```python
from build123d import *

# Parameters (mm, degrees)
SKETCH1_W           = 28
SKETCH1_H           = 78
BOSS_EXTRUDE1_DEPTH = 58
CUT_EXTRUDE1_DEPTH  = 10
CUT_EXTRUDE2_DEPTH  = 20
CUT_EXTRUDE3_DEPTH  = 30
SKETCH5_R           = 2.75
BOSS_EXTRUDE2_DEPTH = 6


with BuildPart() as part:
    # Sketch1 → Boss-Extrude1 (new body)
    with BuildSketch(Plane(origin=(0, 0, 0), x_dir=(1, 0, 0), z_dir=(0, 1, 0))):
        Rectangle(SKETCH1_W, SKETCH1_H)
    extrude(amount=BOSS_EXTRUDE1_DEPTH)

    # Sketch2 → Cut-Extrude1 (cut)
    with BuildSketch(Plane(origin=(14, 0, 0), x_dir=(0, 0, -1), z_dir=(1, 0, 0))):
        Polygon((-39, 8), (-14.181832949, 8), (9.133549959, 58), (-39, 58), align=None)
    extrude(amount=-CUT_EXTRUDE1_DEPTH, mode=Mode.SUBTRACT)

    # Sketch3 → Cut-Extrude2 (cut)
    with BuildSketch(Plane(origin=(4, 0, 0), x_dir=(0, 0, -1), z_dir=(1, 0, 0))):
        Polygon((-39, 16), (-15, 16), (-15, 40.557545824), (1, 40.557545824), (9.133549959, 58), (-39, 58), align=None)
    extrude(amount=-CUT_EXTRUDE2_DEPTH, mode=Mode.SUBTRACT)

    # Sketch4 → Cut-Extrude3 (cut)
    with BuildSketch(Plane(origin=(14, 0, 0), x_dir=(0, 0, -1), z_dir=(1, 0, 0))):
        Polygon((9.133549959, 58), (22.517676281, 52.154545261), (8.109098298, 19.163745323), (12.691153845, 17.162553937), (27.099731828, 50.153353874), (39, 44.95596726), (39, 58), align=None)
    extrude(amount=-CUT_EXTRUDE3_DEPTH, mode=Mode.SUBTRACT)

    # Sketch5 → Boss-Extrude2 (add)
    with BuildSketch(Plane(origin=(0, 52.058969702, -22.736512182), x_dir=(1, 0, 0), z_dir=(0, 0.9164111093707628, -0.40023827730721606))):
        with Locations(Location((-8.021015767, -7.343733433, 0), (0, 0, 90))):
            Circle(SKETCH5_R)
        with Locations(Location((6.818441056, -7.343733433, 0), (0, 0, 90))):
            Circle(SKETCH5_R)
    extrude(amount=BOSS_EXTRUDE2_DEPTH)


solid = part.part
```
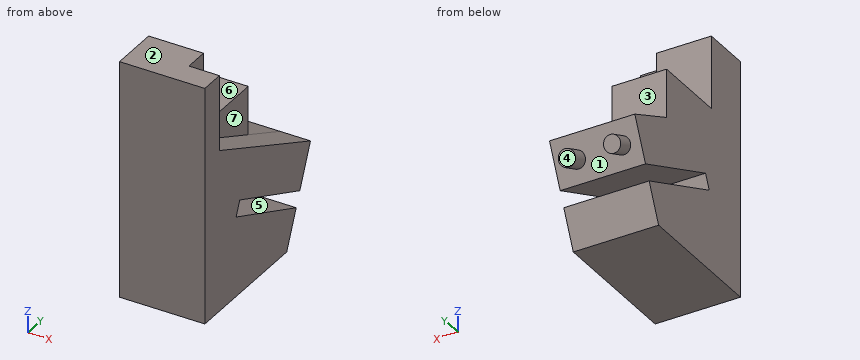
Geometry check sheet. Reference: the model listing, model coordinates, mm. Face numbers are marked on the shaded views. A direction names the side the tool comes from. Coordinates: 2 decimals unless noted, no trailing zeros. Loops run counter-clockwise (first coordinate to the right, second up) from the corner with the lowest first, then second, coordinate; pieces in that order, holes last. Notation, with made-up numbers: (0, -14) - (52, -14) arc R17 cw to (52, -6) - close; hole circle Ø1 at (62.5, -32). An arc over 180 degrees is marked (long way). One line per item, written item: value. Start each with the question number.
(1) Depth check by flat-ended pin: P1, Ø6, axis at x = 9, y = 52, coming from the -Z side; P2, Ø1, axis at x = -2, y = 38, coming from the +Z side; P3, Ø11, axis at x = 8.5, z = 31, coming from the +Y side. Enter the tip coordinate at first touch or a pass-through.
(2) Cross-section at C-C on x = -0.5. Enter the section's corners in (y, z), plus the area to 3 significant figures.
(3) Cross-section at D-D on y = 39. Enter the section's corners in (x, z), plus the area to 3 significant figures.
(4) Mould release check, pull along Z, two halves, no side actions. Record for the marked faces 1, 2, 3 and 4: released by +Z, released by -Z, zero draft, split by the parting line, or undercut.
(5) Cross-section at A-A on z = 20. Enter the section's corners in (x, y), plus the area to 3 significant figures.
(6) Cross-section at B-B on y = 32. Enter the section's corners in (x, z), plus the area to 3 significant figures.
(7) Tool access check on the marked faces 5, 6 and 7. Record the directions out of +Z, -Z, +X, -X, +Y, -Y that give a thin tool (end or side, any length) a straight path to the whole face; none if there is none.
(8) Material ranges on line 1 (Y direction, x = -7, z = 16); line 2 (Z direction, x = 10.25, y = 31); line 3 (Z direction, x = -6.5, y = 19), recorded low to high. Write a range as [from, to].
Results below:
1. P1: stops at z = -29.74
1. P2: stops at z = 15
1. P3: stops at y = 16
2. outline: (0, -39) - (44.96, -39) - (50.15, -27.1) - (17.16, -12.69) - (19.16, -8.11) - (52.15, -22.52) - (58, -9.13) - (40.56, -1) - (40.56, 15) - (16, 15) - (16, 39) - (0, 39) - close
2. area: 2,790 mm2
3. outline: (-14, -39) - (14, -39) - (14, -22.23) - (-14, -22.23) - close; (-14, -16.77) - (14, -16.77) - (14, -0.27) - (4, -0.27) - (4, 15) - (-14, 15) - close
3. area: 1,210 mm2
4. face 1: undercut
4. face 2: released by +Z
4. face 3: zero draft
4. face 4: released by -Z
5. outline: (-14, 0) - (14, 0) - (14, 8) - (4, 8) - (4, 16) - (-14, 16) - close
5. area: 368 mm2
6. outline: (-14, -39) - (14, -39) - (14, -19.17) - (-14, -19.17) - close; (-14, -13.72) - (14, -13.72) - (14, 2.99) - (4, 2.99) - (4, 15) - (-14, 15) - close
6. area: 1,240 mm2
7. face 5: +X, -X
7. face 6: +Z, +X, -X, +Y
7. face 7: +Z, +X, +Y
8. line 1: y = [0, 16]
8. line 2: z = [-39, -18.73], [-13.28, 3.46]
8. line 3: z = [-39, -13.49], [-8.48, 15]
